Source: CAD feature listing. Evaluate the final solid. Frame: model axes, mm. Give positions to 0.01 mm unless a question says otherwise; leave off trailing zeros. Write each loop counter-clockwise with the first axis right and the second up, starting at its lowest first coordinate (ties: lowest second). Pieces come first, ordered by that corner, then holes.
```python
from build123d import *

# Parameters (mm, degrees)
BOSS_EXTRUDE1_DEPTH = 60
SKETCH2_W           = 26
SKETCH2_H           = 30
BOSS_EXTRUDE2_DEPTH = 60


with BuildPart() as part:
    # Sketch1 → Boss-Extrude1 (new body)
    with BuildSketch(Plane(origin=(0, 0, 0), x_dir=(0, 0, -1), z_dir=(1, 0, 0))):
        Polygon((0, 0), (-59.234177215, 375.354915047), (-33.234177215, 375.354915047), (105, 0), align=None)
    extrude(amount=BOSS_EXTRUDE1_DEPTH)

    # Sketch2 → Boss-Extrude2 (add)
    with BuildSketch(Plane.ZY):
        with Locations((46.234177215, 360.354915047)):
            Rectangle(SKETCH2_W, SKETCH2_H)
    extrude(amount=-BOSS_EXTRUDE2_DEPTH)


solid = part.part
```
1. Section query B-B (y = 205). Return loops of the section in (x, z).
2. Pin query (flat end, axial travel): P1, Ø10, axis at x = 12, y = 118.5, coming from the -Z side; P2, Ø1, axis at x = 43.5, y = 241.5, coming from the -Z side; P3, Ø1.4, axis at x = 15, z = 57.5, coming from the -Y side. Return the tip coordinate at first contact, or that it passes through.
3. Line query: probe 1 along Z at (x, y) = (51.5, 245.5); probe 2 along Z at (x, y) = (29, 109.5). Output: solid intervals per line, ascending.
4. Section query A-A (x = 25.5). Return loops of the section in (y, z), plus the area to 3 significant figures.
5. Section query C-C (z = -34). Return loops of the section in (x, y).
The answers:
1. outline: (0, -29.5) - (60, -29.5) - (60, 32.35) - (0, 32.35) - close
2. P1: stops at z = -63.2
2. P2: stops at z = -16.25
2. P3: stops at y = 345.35
3. probe 1: z = -14.59 to 38.74
3. probe 2: z = -64.67 to 17.28
4. outline: (0, -105) - (375.35, 33.23) - (375.35, 59.23) - (345.35, 59.23) - (345.35, 54.5) - (0, 0) - close
4. area: 24,700 mm2
5. outline: (0, 0) - (60, 0) - (60, 192.79) - (0, 192.79) - close
